Part print with two shaded views. Sizes in mm from the minimum x, y, z corner. A direction names the side the tool comes from. Coordinates: 2 decimals unless noted, no trailing zeros. Order: outer loops, then holes, each group sorted by start corner. A loop starts at its lowest first (then second) coordinate and runs counter-clockwise, first axis right, second up. Notation, with made-up numbers: (46.25, 9) - (83.25, 9) arc R15 cw to (83.25, 37) - close; hole circle Ø4 at (41.25, 69). An arc over 180 degrees is marked (long way). Return JSON: item names as keys, results as strings.
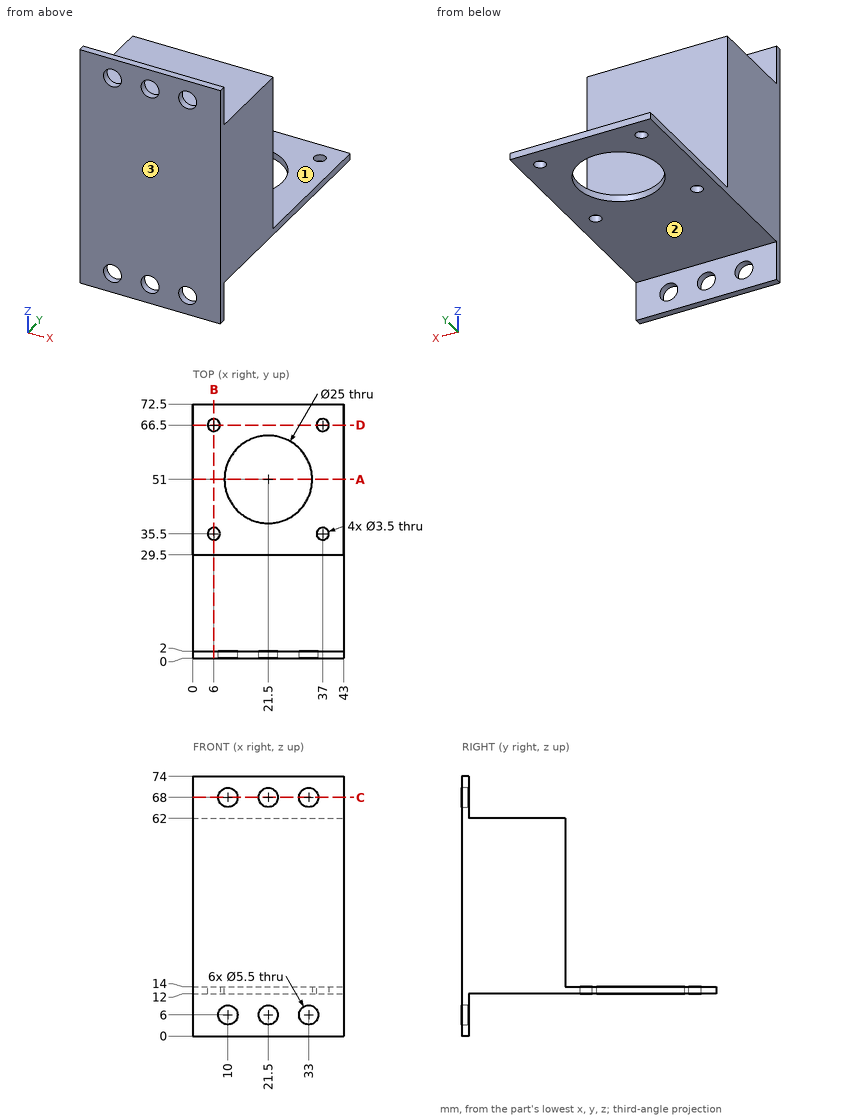
Item 1: Which spindle directions (+Z, -Z, +X, -X, +Y, -Y) get a long thin tool onto all of the face, cutting with end or side? Do the marked faces 1, 2 and 3. Say none if no direction does.
Findings below:
{"face 1": "+Z, +X, -X, +Y", "face 2": "-Z, +X, -X, +Y", "face 3": "+Z, -Z, +X, -X, -Y"}
Item 2: Band-saw the part on B-B, the plane x = 6. List the corners of the cut face in (y, z), then the cut area to 4 significant figures.
Findings below:
{"outline": "(0, 0) - (2, 0) - (2, 12) - (33.75, 12) - (33.75, 14) - (29.5, 14) - (29.5, 62) - (2, 62) - (2, 74) - (0, 74) - close; (37.25, 12) - (64.75, 12) - (64.75, 14) - (37.25, 14) - close; (68.25, 12) - (72.5, 12) - (72.5, 14) - (68.25, 14) - close", "area": "1,595 mm²"}
Item 3: Band-saw the part on A-A, the plane y = 51. List the corners of the cut face in (x, z), then the cut area to 3 significant figures.
Findings below:
{"outline": "(0, 12) - (9, 12) - (9, 14) - (0, 14) - close; (34, 12) - (43, 12) - (43, 14) - (34, 14) - close", "area": "36.0 mm²"}
Item 4: Drop flat-ended pins along their axis: P1, Ø4, axis at x = 13.5, y = 24.5, coming from the +Z side; P2, Ø8, axis at x = 19.5, y = 60, coming from the +Z side; P3, Ø9, axis at x = 33, z = 68, coming from the +Y side; P4, Ø4.5, axis at x = 21.5, z = 6, coming from the +Y side. Give the stop position or say it passes through.
Findings below:
{"P1": "stops at z = 62", "P2": "stops at z = 14", "P3": "stops at y = 2", "P4": "passes through"}
Item 5: Band-saw the part on C-C, the plane z = 68. List the corners of the cut face in (x, y).
Findings below:
{"outline": "(0, 0) - (7.25, 0) - (7.25, 2) - (0, 2) - close; (12.75, 0) - (18.75, 0) - (18.75, 2) - (12.75, 2) - close; (24.25, 0) - (30.25, 0) - (30.25, 2) - (24.25, 2) - close; (35.75, 0) - (43, 0) - (43, 2) - (35.75, 2) - close"}
Item 6: Wall check: L1, parallel to X at y = 0.85, z = 68; L2, parallel to Y at x = 6, z = 12.75; L3, parallel to X at y = 35, z = 13. Give the ranges that are in metal, low to high. Write a range as [from, to].
Findings below:
{"L1": "x = [0, 7.25], [12.75, 18.75], [24.25, 30.25], [35.75, 43]", "L2": "y = [0, 33.75], [37.25, 64.75], [68.25, 72.5]", "L3": "x = [0, 4.32], [7.68, 35.32], [38.68, 43]"}
Item 7: Band-saw the part on D-D, the plane y = 66.5. List the corners of the cut face in (x, z).
Findings below:
{"outline": "(0, 12) - (4.25, 12) - (4.25, 14) - (0, 14) - close; (7.75, 12) - (35.25, 12) - (35.25, 14) - (7.75, 14) - close; (38.75, 12) - (43, 12) - (43, 14) - (38.75, 14) - close"}
